from build123d import *

# Parameters (mm, degrees)
SKETCH2_W           = 80
SKETCH2_H           = 30
BOSS_EXTRUDE1_DEPTH = 4
SKETCH3_R           = 1.75
CUT_EXTRUDE1_DEPTH  = 5


with BuildPart() as part:
    # Sketch2 → Boss-Extrude1 (new body)
    with BuildSketch(Plane(origin=(0, 0, 0), x_dir=(1, 0, 0), z_dir=(0, 1, 0))):
        with Locations((40, 15)):
            Rectangle(SKETCH2_W, SKETCH2_H)
    extrude(amount=BOSS_EXTRUDE1_DEPTH)

    # Sketch3 → Cut-Extrude1 (cut, through all)
    with BuildSketch(Plane(origin=(0, 4, 0), x_dir=(1, 0, 0), z_dir=(0, 1, 0))):
        with Locations((6, 6)):
            Circle(SKETCH3_R)
        with Locations((6, 24)):
            Circle(SKETCH3_R)
        with Locations((74, 24)):
            Circle(SKETCH3_R)
        with Locations((74, 6)):
            Circle(SKETCH3_R)
        with BuildLine():
            Line((13.95, 0), (26.05, 0))
            Line((26.05, 0), (26.05, 15))
            ThreePointArc((26.05, 15), (20, 21.05), (13.95, 15))
            Line((13.95, 15), (13.95, 0))
        make_face()
        with BuildLine():
            Line((53.95, 30), (53.95, 15))
            ThreePointArc((53.95, 15), (60, 8.95), (66.05, 15))
            Line((66.05, 15), (66.05, 30))
            Line((66.05, 30), (53.95, 30))
        make_face()
    extrude(amount=-CUT_EXTRUDE1_DEPTH, mode=Mode.SUBTRACT)


solid = part.part
Work out the finished part from the listing and answer in its coordinate system (mm). A direction names the side the tool comes from. Coordinates: 2 decimals unless noted, no trailing zeros. Loops run counter-clockwise (first coordinate to the right, second up) from the corner with the lowest first, then second, coordinate; pieces in that order, holes last. Notation, with made-up numbers: (73, -17.75) -> (112, -17.75) arc R14 ccw to (112, 0.25) -> close; hole circle Ø3 at (89.5, 74.25). An arc over 180 degrees is marked (long way). Write each question's results on one line, items separated by ' | '. Start each with the question number.
1) Consider line 1 along X through (y, z) = (2.85, -24); line 2 along Z through (x, y) = (74, 1.7); line 3 along X through (y, z) = (2.7, -1.75). Determine where each line is inside the solid, lowest interval first.
2) The mould has two halves that part along X. Classify faces 4 (the flat face through (0, 2, -15)), 5 (the flat face through (39, 0, -15)), 6 (the flat face through (53.95, 2, -23)): pulls with the +X half, pulls with the -X half, needs draft (parallel to the pull), parting line crosses it, or undercut.
3) For faces 1 (the flat face through (26.05, 2, -7)), 2 (the cylindrical face through (5.772, 2.028, -25.735)), 3 (the flat face through (66.05, 2, -22)), determine the directions among +Z, -Z, +X, -X, +Y, -Y from which every point of the face is accessible in a straight line to the end or side of a thin tool.
4) Find section A-A on z = -24. Determine the outline of the cut face in (x, y).
5) Find section B-B on x = 6. Determine the outline of the cut face in (y, z).
6) Find section D-D on z = -16. Determine the outline of the cut face in (x, y), then the cut area to 3 significant figures.
7) Flat-ended cylindrical pins translate along their axes: P1, Ø2, axis at y = 2, z = -11, coming from the -X side; P2, Ø1.5, axis at x = 15, z = -15.5, coming from the +Y side. Find the tip coordinate at first contact, or state that the pin passes through.
8) Find section C-C on y = 2.9. Determine the outline of the cut face in (x, z).
Response values:
1) line 1: x = 0 to 4.25, 7.75 to 53.95, 66.05 to 72.25, 75.75 to 80 | line 2: z = -30 to -25.75, -22.25 to -7.75, -4.25 to 0 | line 3: x = 0 to 13.95, 26.05 to 80
2) face 4: pulls with the -X half | face 5: needs draft | face 6: undercut
3) face 1: +Z, +Y, -Y | face 2: +Y, -Y | face 3: -Z, +Y, -Y
4) outline: (0, 0) -> (4.25, 0) -> (4.25, 4) -> (0, 4) -> close; (7.75, 0) -> (53.95, 0) -> (53.95, 4) -> (7.75, 4) -> close; (66.05, 0) -> (72.25, 0) -> (72.25, 4) -> (66.05, 4) -> close; (75.75, 0) -> (80, 0) -> (80, 4) -> (75.75, 4) -> close
5) outline: (0, -30) -> (4, -30) -> (4, -25.75) -> (0, -25.75) -> close; (0, -22.25) -> (4, -22.25) -> (4, -7.75) -> (0, -7.75) -> close; (0, -4.25) -> (4, -4.25) -> (4, 0) -> (0, 0) -> close
6) outline: (0, 0) -> (14.03, 0) -> (14.03, 4) -> (0, 4) -> close; (25.97, 0) -> (53.95, 0) -> (53.95, 4) -> (25.97, 4) -> close; (66.05, 0) -> (80, 0) -> (80, 4) -> (66.05, 4) -> close | area: 224 mm^2
7) P1: stops at x = 0 | P2: passes through
8) outline: (0, -30) -> (53.95, -30) -> (53.95, -15) arc R6.05 cw to (66.05, -15) -> (66.05, -30) -> (80, -30) -> (80, 0) -> (26.05, 0) -> (26.05, -15) arc R6.05 cw to (13.95, -15) -> (13.95, 0) -> (0, 0) -> close; hole circle Ø3.5 at (6, -24); hole circle Ø3.5 at (6, -6); hole circle Ø3.5 at (74, -24); hole circle Ø3.5 at (74, -6)
